Input: part model. Units: mm. Frame: model coordinates. A direction names the side the tool comes from. Coordinates: 2 decimals unless noted, no trailing zeros. Order: outer loops, then holes, each group sorted by start corner. A loop starts at its lowest first (then second) coordinate and runs counter-clockwise, first axis right, second up. Notation, with made-up numbers: (35.25, -5.75) - (86.25, -5.75) arc R21 ccw to (86.25, 7.25) - close; hole circle Ø1 at (-16.5, 30). An arc over 180 degrees is marked (long way). One line per question, with ' | ' between items. Start each with the question number.
```python
from build123d import *

# Parameters (mm, degrees)
SKETCH1_R           = 1.5875
BOSS_EXTRUDE1_DEPTH = 3


with BuildPart() as part:
    # Sketch1 → Boss-Extrude1 (new body)
    with BuildSketch(Plane.XY):
        with BuildLine():
            Line((48, 140), (24, 140))
            Line((24, 140), (24, 143))
            Line((24, 143), (-3, 143))
            Line((-3, 143), (-3, 140))
            Line((-3, 140), (0, 140))
            Line((0, 140), (0, 112))
            Line((0, 112), (-3, 112))
            Line((-3, 112), (-3, 84))
            Line((-3, 84), (0, 84))
            Line((0, 84), (0, 80.091592476))
            Line((0, 80.091592476), (9.204842615, 80.091592476))
            ThreePointArc((9.204842615, 80.091592476), (10.844002051, 79.815272857), (12.301988723, 79.016855013))
            ThreePointArc((12.301988723, 79.016855013), (16.805573917, 89.764144743), (24.1194552, 98.835729872))
            Line((24.1194552, 98.835729872), (21.793869689, 98.835729872))
            ThreePointArc((21.793869689, 98.835729872), (18.258335784, 100.300195966), (16.793869689, 103.835729872))
            Line((16.793869689, 103.835729872), (16.793869689, 112.604597993))
            ThreePointArc((16.793869689, 112.604597993), (18.258335784, 116.140131899), (21.793869689, 117.604597993))
            Line((21.793869689, 117.604597993), (38.117364989, 117.604597993))
            ThreePointArc((38.117364989, 117.604597993), (41.652898895, 116.140131899), (43.117364989, 112.604597993))
            Line((43.117364989, 112.604597993), (43.117364989, 108.94733597))
            ThreePointArc((43.117364989, 108.94733597), (58.575877607, 109.555709088), (73.183096051, 104.460132622))
            Line((73.183096051, 104.460132622), (73.183096051, 112.523924668))
            ThreePointArc((73.183096051, 112.523924668), (74.647562145, 116.059458574), (78.183096051, 117.523924668))
            Line((78.183096051, 117.523924668), (88.946846839, 117.523924668))
            ThreePointArc((88.946846839, 117.523924668), (92.482380745, 116.059458574), (93.946846839, 112.523924668))
            Line((93.946846839, 112.523924668), (93.946846839, 96.632091269))
            ThreePointArc((93.946846839, 96.632091269), (92.482380745, 93.096557363), (88.946846839, 91.632091269))
            Line((88.946846839, 91.632091269), (86.912064447, 91.632091269))
            ThreePointArc((86.912064447, 91.632091269), (93.547360155, 62.743436939), (79.217418381, 36.796678628))
            Line((79.217418381, 36.796678628), (80.114705661, 36.796678628))
            ThreePointArc((80.114705661, 36.796678628), (83.650239567, 35.332212534), (85.114705661, 31.796678628))
            Line((85.114705661, 31.796678628), (85.114705661, 26.165851447))
            ThreePointArc((85.114705661, 26.165851447), (83.650239567, 22.630317541), (80.114705661, 21.165851447))
            Line((80.114705661, 21.165851447), (65.40791431, 21.165851447))
            ThreePointArc((65.40791431, 21.165851447), (62.555840914, 22.059067139), (60.722774204, 24.419580508))
            Line((60.722774204, 24.419580508), (55.609195041, 15.562601589))
            ThreePointArc((55.609195041, 15.562601589), (53.114505039, 13.411669321), (49.823236264, 13.279239393))
            ThreePointArc((49.823236264, 13.279239393), (27.558248735, 5.305071401), (23.135588282, 28.537744501))
            Line((23.135588282, 28.537744501), (19.764061802, 30.484296222))
            ThreePointArc((19.764061802, 30.484296222), (17.434432671, 33.520328015), (17.933934783, 37.314423241))
            Line((17.933934783, 37.314423241), (20.590822265, 41.91628735))
            ThreePointArc((20.590822265, 41.91628735), (15.836008812, 48.974059185), (12.620809049, 56.853328488))
            ThreePointArc((12.620809049, 56.853328488), (11.041151458, 55.853928303), (9.204842615, 55.50451642))
            Line((9.204842615, 55.50451642), (-3, 55.50451642))
            Line((-3, 55.50451642), (-3, 28))
            Line((-3, 28), (0, 28))
            Line((0, 28), (0, 0))
            Line((0, 0), (-3, 0))
            Line((-3, 0), (-3, -3))
            Line((-3, -3), (24, -3))
            Line((24, -3), (24, 0))
            Line((24, 0), (48, 0))
            Line((48, 0), (48, -3))
            Line((48, -3), (72, -3))
            Line((72, -3), (72, 0))
            Line((72, 0), (96, 0))
            Line((96, 0), (96, -3))
            Line((96, -3), (123, -3))
            Line((123, -3), (123, 0))
            Line((123, 0), (120, 0))
            Line((120, 0), (120, 28))
            Line((120, 28), (123, 28))
            Line((123, 28), (123, 56))
            Line((123, 56), (120, 56))
            Line((120, 56), (120, 84))
            Line((120, 84), (123, 84))
            Line((123, 84), (123, 112))
            Line((123, 112), (120, 112))
            Line((120, 112), (120, 140))
            Line((120, 140), (123, 140))
            Line((123, 140), (123, 143))
            Line((123, 143), (96, 143))
            Line((96, 143), (96, 140))
            Line((96, 140), (72, 140))
            Line((72, 140), (72, 143))
            Line((72, 143), (48, 143))
            Line((48, 143), (48, 140))
        make_face()
        with Locations((7.111536912, 17.559834216)):
            Circle(SKETCH1_R, mode=Mode.SUBTRACT)
        with BuildLine():
            ThreePointArc((11.493043158, 14.559834216), (11.846596549, 14.413387607), (11.993043158, 14.059834216))
            Line((11.993043158, 14.059834216), (11.993043158, 12.498677253))
            ThreePointArc((11.993043158, 12.498677253), (11.846596549, 12.145123862), (11.493043158, 11.998677253))
            Line((11.493043158, 11.998677253), (3.35499228, 11.998677253))
            ThreePointArc((3.35499228, 11.998677253), (1.940778717, 12.58446369), (1.35499228, 13.998677253))
            Line((1.35499228, 13.998677253), (1.35499228, 24.79117874))
            ThreePointArc((1.35499228, 24.79117874), (1.501964385, 25.145256847), (1.856477503, 25.291176534))
            Line((1.856477503, 25.291176534), (3.613022136, 25.285958787))
            ThreePointArc((3.613022136, 25.285958787), (3.965615019, 25.138988887), (4.111536912, 24.785960993))
            Line((4.111536912, 24.785960993), (4.111536912, 17.559834216))
            ThreePointArc((4.111536912, 17.559834216), (4.990216569, 15.438513872), (7.111536912, 14.559834216))
            Line((7.111536912, 14.559834216), (11.493043158, 14.559834216))
        make_face(mode=Mode.SUBTRACT)
        with Locations((102.35, 27.6)):
            Circle(SKETCH1_R, mode=Mode.SUBTRACT)
        with Locations((7.25, 117.4)):
            Circle(SKETCH1_R, mode=Mode.SUBTRACT)
        with Locations((102.35, 107.5)):
            Circle(SKETCH1_R, mode=Mode.SUBTRACT)
    extrude(amount=BOSS_EXTRUDE1_DEPTH)


solid = part.part
```
(1) Section C-C (x = 29.5). Output: boundary loops of the cut face in (y, z).
(2) Section A-A (x = 102.35). Output: boundary loops of the cut face in (y, z), then the cut area to 3 significant figures.
(3) Section B-B (y = 89). Output: boundary loops of the cut face in (x, z).
(4) Draft query along X for faces 6 (the face through (16.794, 108, 1)), 7 (the face through (110, 143, 1)), 8 (the face through (-3, 142, 1)), 9 (the face through (123, 98, 1)). Return one class per face: +X half, -X half, draft (parallel to the pull), parting line (faces both ways), or undercut.
(5) Reachability of faces 1 (the face through (24, -2, 1)), 2 (the face through (30, 117.605, 1)), 3 (the face through (121, 140, 1)), 4 (the face through (60, 143, 1)), 5 (the face through (0, 82, 1)) from +Z, -Z, +X, -X, +Y, -Y: full face, straight path, thin tool, end or side. Return the list, or none.
(6) Pin query (flat end, axial travel): pin 1 (0.9 mm diameter, centred on y = 21.5, z = 1.5, fed in from +X); pin 2 (1.6 mm diameter, centred on x = 88, z = 2, fed in from +Y); pin 3 (0.5 mm diameter, centred on y = 13, z = 1.5, fed in from -X). Return the tip coordinate at first contact, or that it passes through.
(7) Material intervals for line 1 along X through (y, z) = (111, 1.85); line 2 along Y through (x, z) = (7.25, 0.8); line 3 along X through (y, z) = (25, 1.55), sorted ascending. Write a range as from..to.
(8) Section D-D (y = 130). Output: boundary loops of the cut face in (x, z), then the cut area to 3 significant figures.
Worked answers:
1) outline: (0, 0) - (4.37, 0) - (4.37, 3) - (0, 3) - close; (117.6, 0) - (140, 0) - (140, 3) - (117.6, 3) - close
2) outline: (-3, 0) - (26.01, 0) - (26.01, 3) - (-3, 3) - close; (29.19, 0) - (105.91, 0) - (105.91, 3) - (29.19, 3) - close; (109.09, 0) - (143, 0) - (143, 3) - (109.09, 3) - close | area: 419 mm²
3) outline: (-3, 0) - (16.36, 0) - (16.36, 3) - (-3, 3) - close; (88.54, 0) - (123, 0) - (123, 3) - (88.54, 3) - close
4) face 6: undercut | face 7: draft | face 8: -X half | face 9: +X half
5) face 1: +Z, -Z, -Y | face 2: +Z, -Z | face 3: +Z, -Z, +X | face 4: +Z, -Z, +X, -X, +Y | face 5: +Z, -Z, -X
6) pin 1: stops at x = 120 | pin 2: stops at y = 140 | pin 3: stops at x = 0
7) line 1: x = -3..16.79, 43.12..73.18, 93.95..123 | line 2: y = -3..12, 14.56..15.98, 19.14..55.5, 80.09..115.81, 118.99..143 | line 3: x = 0..1.4, 4.06..21, 84.98..120
8) outline: (0, 0) - (120, 0) - (120, 3) - (0, 3) - close | area: 360 mm²
